Source: CAD feature listing. Evaluate the final solid. Frame: model axes, mm. A direction names the side the tool comes from. Round coordinates to 2 decimals unless told otherwise and drop trailing zeros. Write each loop counter-clockwise with the first axis right and the second up, starting at its lowest first coordinate (ties: lowest second). Pieces come first, ordered by that corner, then holes. Notation, with made-up numbers: (57.25, 17) -> (82.25, 17) arc R13 ccw to (82.25, 33) -> close; hole circle Ø1 at (-27, 74.5). An arc over 180 degrees is marked (long way). Return JSON: item names as keys, results as strings. Group by question number.
from build123d import *

# Parameters (mm, degrees)
SKETCH_1_W               = 36
SKETCH_1_H               = 30
EXTRUDE_1_DEPTH          = 5
SKETCH_4_W               = 33
SKETCH_4_H               = 12
CUT_EXTRUDE_2_DEPTH      = 2
SKETCH_8_R               = 1
CUT_EXTRUDE_6_DEPTH      = 3
CUT_EXTRUDE_3_DEPTH      = 24.622023622
CUT_EXTRUDE_3_DEPTH_BACK = 3
SKETCH_5_W               = 23.5
SKETCH_5_H               = 12
SKETCH_9_R               = 1
CUT_EXTRUDE_7_DEPTH      = 5
SKETCH_11_W              = 15
SKETCH_11_H              = 5
EXTRUDE_3_DEPTH          = 25
CUT_EXTRUDE_8_REACH      = 45
SKETCH_12_R              = 3


with BuildPart() as part:
    # 草图1 → 凸台-拉伸1 (new body)
    with BuildSketch(Plane(origin=(0, 0, 0), x_dir=(1, 0, 0), z_dir=(0, 1, 0))):
        Rectangle(SKETCH_1_W, SKETCH_1_H)
    extrude(amount=EXTRUDE_1_DEPTH)

    # 草图4 → 切除-拉伸2 (cut)
    with BuildSketch(Plane.XZ):
        Rectangle(SKETCH_4_W, SKETCH_4_H)
    extrude(amount=-CUT_EXTRUDE_2_DEPTH, mode=Mode.SUBTRACT)

    # 草图8 → 切除-拉伸6 (cut)
    with BuildSketch(Plane.XZ.offset(-2)):
        with Locations(Location((14, 0, 0), (0, 0, 270))):
            Circle(SKETCH_8_R)
        with Locations(Location((-14, 0, 0), (0, 0, 270))):
            Circle(SKETCH_8_R)
    extrude(amount=-CUT_EXTRUDE_6_DEPTH, mode=Mode.SUBTRACT)

    # 草图5 → 切除-拉伸3 (cut, two sides: drawn at the far end of the back side and taken through both)
    with BuildSketch(Plane.XZ.offset(-2).offset(-CUT_EXTRUDE_3_DEPTH_BACK)):
        Rectangle(SKETCH_5_W, SKETCH_5_H)
    extrude(amount=CUT_EXTRUDE_3_DEPTH + CUT_EXTRUDE_3_DEPTH_BACK, mode=Mode.SUBTRACT)

    # 草图9 → 切除-拉伸7 (cut)
    with BuildSketch(Plane(origin=(0, 0, -15), x_dir=(-1, 0, 0), z_dir=(0, 0, -1))):
        with Locations((12, 2.5)):
            Circle(SKETCH_9_R)
        with Locations(Location((-12, 2.5, 0), (0, 0, 180))):
            Circle(SKETCH_9_R)
    cut_extrude_7 = extrude(amount=-CUT_EXTRUDE_7_DEPTH, mode=Mode.SUBTRACT)

    # 镜向1: 切除-拉伸7 across plane
    add(cut_extrude_7.mirror(Plane.XY), mode=Mode.SUBTRACT)

    # 草图11 → 凸台-拉伸3 (add)
    with BuildSketch(Plane.XZ):
        with Locations((0, 12.5)):
            Rectangle(SKETCH_11_W, SKETCH_11_H)
        with Locations((0, -12.5)):
            Rectangle(SKETCH_11_W, SKETCH_11_H)
    extrude(amount=EXTRUDE_3_DEPTH)

    # 切除-拉伸8: up to this face of the body (flat: up to its plane)
    cut_extrude_8_end = Plane(part.part.faces().sort_by_distance((0, -7.75118941, 15))[0])
    # 草图12 → 切除-拉伸8 (cut, up to the picked face)
    with BuildSketch(Plane(origin=(0, 0, -15), x_dir=(-1, 0, 0), z_dir=(0, 0, -1)), mode=Mode.PRIVATE) as cut_extrude_8_sk1:
        with Locations((0, -20)):
            Circle(SKETCH_12_R)
    cut_extrude_8_tool1 = split(extrude(cut_extrude_8_sk1.sketch, amount=-CUT_EXTRUDE_8_REACH, mode=Mode.PRIVATE), bisect_by=cut_extrude_8_end, keep=Keep.BOTH, mode=Mode.PRIVATE)
    add(cut_extrude_8_tool1.solids().sort_by(Axis((0, -20, -15), (0, 0, 1)))[0], mode=Mode.SUBTRACT)


solid = part.part
Item 1: Material intervals for probe 1 along X at (y, z) = (3.1, 0); probe 2 along Z at (x, y) = (-2.5, -13.75); probe 3 along Z at (x, y) = (7.5, 2), sorted ascending.
Item 2: Cut plane A-A on y = -5. Output: boundary loops of the cut face in (x, z), and give its area (3 significant figures).
Item 3: Cut plane D-D on y = -20. Output: boundary loops of the cut face in (x, z), and give its area (3 significant figures).
Item 4: Cut plane C-C on x = -4. Output: boundary loops of the cut face in (y, z).
Item 5: Pull-direction query (Y, two-part tool) for faces 1 (the cylindrical face through (0.65, -22.93, -12.54)), 2 (the flat face through (18, 2, 0)), 3 (the flat face through (0, 5, -7)); classes: +Y half, -Y half, draft (parallel to the pull), parting line (faces both ways), or undercut.
Item 6: Cut plane B-B on z = -1.75. Output: boundary loops of the cut face in (x, y), and give its area (3 significant figures).
Item 7: First-contact query: pin 1 Ø5.5 at (x, y) = (0, -20) entering from +Z; pin 2 Ø2.5 at (x, z) = (14, 0) entering from -Y; pin 3 Ø2.5 at (y, z) = (-12.5, 12.5) entering from +X; pin 4 Ø0.6 at (x, y) = (-12, 3) entering from -Z. Flat tips, straight axial feed; report the tip coordinate or a pass-through.
Item 8: Set-up query: faces 4 (the flat face through (-7.5, -12, -13)), 5 (the cylindrical face through (-11, 2.5, 12.5)), 6 (the cylindrical face through (-11, 2.5, -12.5)), 7 (the flat face through (11.75, 4, 0)), 8 (the flat face through (-15.2, 2, 0.1)). Return all of +Z, -Z, +X, -X, +Y, -Y with unobstructed straight access to the full face (end or side cutting, diameter ignored); none if empty.
Here are the results:
{
 "1": {"probe 1": "x = -18 to -15, -13 to -11.75, 11.75 to 13, 15 to 18", "probe 2": "z = -15 to -10, 10 to 15", "probe 3": "z = -15 to -6, 6 to 15"},
 "2": {"outline": "(-7.5, -15) -> (7.5, -15) -> (7.5, -10) -> (-7.5, -10) -> close; (-7.5, 10) -> (7.5, 10) -> (7.5, 15) -> (-7.5, 15) -> close", "area": "150 mm^2"},
 "3": {"outline": "(-7.5, -15) -> (-3, -15) -> (-3, -10) -> (-7.5, -10) -> close; (-7.5, 10) -> (-3, 10) -> (-3, 15) -> (-7.5, 15) -> close; (3, -15) -> (7.5, -15) -> (7.5, -10) -> (3, -10) -> close; (3, 10) -> (7.5, 10) -> (7.5, 15) -> (3, 15) -> close", "area": "90.0 mm^2"},
 "4": {"outline": "(-25, -15) -> (5, -15) -> (5, -6) -> (0, -6) -> (0, -10) -> (-25, -10) -> close; (-25, 10) -> (0, 10) -> (0, 6) -> (5, 6) -> (5, 15) -> (-25, 15) -> close"},
 "5": {"face 1": "undercut", "face 2": "draft", "face 3": "+Y half"},
 "6": {"outline": "(-18, 0) -> (-16.5, 0) -> (-16.5, 2) -> (-11.75, 2) -> (-11.75, 5) -> (-18, 5) -> close; (11.75, 2) -> (16.5, 2) -> (16.5, 0) -> (18, 0) -> (18, 5) -> (11.75, 5) -> close", "area": "43.5 mm^2"},
 "7": {"pin 1": "passes through", "pin 2": "stops at y = 2", "pin 3": "stops at x = 7.5", "pin 4": "stops at z = -10"},
 "8": {"face 4": "+Z, -Z, -X, -Y", "face 5": "+Z", "face 6": "-Z", "face 7": "+Y, -Y", "face 8": "-Y"}
}
